Geometry: final body of the model. Coordinates: model frame, mm. A direction names the side the tool comes from. Give positions to 0.01 mm unless a question says otherwise; leave off trailing zeros. Write each loop counter-clockwise with the first axis right and the second up, starting at its lowest first coordinate (ties: lowest second). Pieces come first, ordered by that corner, then holes. Notation, with made-up numbers: (19, 4) -> (70, 4) arc R27 cw to (70, 38) -> close; hole circle Ø3 at (33.25, 59). An arc over 180 degrees is marked (long way). Answer in a Markdown table with one row per item. Add a question column.
from build123d import *

# Parameters (mm, degrees)
F0_R     = 1.5
F1_DEPTH = 5
F2_R     = 5


# Not quite as in the source:
# - a feature names something its author has since deleted; it is built from what else it names


with BuildPart() as f1:
    # F0 (on Top) → F1 (new body)
    with BuildSketch(Plane.XY):
        with BuildLine():
            Line((32, -25.9806431703), (45.0002060157, -25.9806431703))
            Line((45.0002060157, -25.9806431703), (34.8648160141, -8.425632733))
            ThreePointArc((34.8648160141, -8.425632733), (33.2306953855, -12.3086021935), (31.1657699329, -15.9806431703))
            Line((31.1657699329, -15.9806431703), (32, -15.9806431703))
            Line((32, -15.9806431703), (32, -25.9806431703))
        make_face()
        with BuildLine():
            Line((34.8648160141, -8.425632733), (45.0002060157, -25.9806431703))
            ThreePointArc((45.0002060157, -25.9806431703), (42.4187903028, 24.4905), (0.0002060157, 51.9616431703))
            Line((0.0002060157, 51.9616431703), (6.7047123911, 40.3490974884))
            ThreePointArc((6.7047123911, 40.3490974884), (28.4347881869, 27.6357391565), (37, 3.9616431703))
            ThreePointArc((37, 3.9616431703), (36.4622969142, -2.3233312719), (34.8648160141, -8.425632733))
        make_face()
        with Locations((41.2026322213, 9.0961922878)):
            Circle(F0_R, mode=Mode.SUBTRACT)
        with Locations((25.2027902051, 36.8090964203)):
            Circle(F0_R, mode=Mode.SUBTRACT)
        with BuildLine():
            Line((32, -55.9806431703), (32, -25.9806431703))
            Line((32, -25.9806431703), (21.7361332508, -25.9806431703))
            ThreePointArc((21.7361332508, -25.9806431703), (0, -33.0383568297), (-21.7361332508, -25.9806431703))
            Line((-21.7361332508, -25.9806431703), (-32, -25.9806431703))
            Line((-32, -25.9806431703), (-32, -55.9806431703))
            Line((-32, -55.9806431703), (32, -55.9806431703))
        make_face()
        with Locations((-16, -50.8592247836)):
            Circle(F0_R, mode=Mode.SUBTRACT)
        with Locations((-24.9, -29.9806431703)):
            Circle(F0_R, mode=Mode.SUBTRACT)
        with Locations((16, -50.9806431703)):
            Circle(F0_R, mode=Mode.SUBTRACT)
        with Locations((24.9, -29.9806431703)):
            Circle(F0_R, mode=Mode.SUBTRACT)
        with BuildLine():
            Line((21.7361332508, -25.9806431703), (32, -25.9806431703))
            Line((32, -25.9806431703), (32, -15.9806431703))
            Line((32, -15.9806431703), (31.1657699329, -15.9806431703))
            ThreePointArc((31.1657699329, -15.9806431703), (26.9193766665, -21.422350997), (21.7361332508, -25.9806431703))
        make_face()
        with BuildLine():
            Line((6.7047123911, 40.3490974884), (0.0002060157, 51.9616431703))
            Line((0.0002060157, 51.9616431703), (-6.7042513108, 40.3491824435))
            ThreePointArc((-6.7042513108, 40.3491824435), (0.0002344208, 40.9616431696), (6.7047123911, 40.3490974884))
        make_face()
        with BuildLine():
            Line((-6.7042513108, 40.3491824435), (0.0002060157, 51.9616431703))
            ThreePointArc((0.0002060157, 51.9616431703), (-42.4183782713, 24.4905), (-44.9997939843, -25.9806431703))
            Line((-44.9997939843, -25.9806431703), (-34.8646590472, -8.4260745178))
            ThreePointArc((-34.8646590472, -8.4260745178), (-32.04293994, 22.4616431703), (-6.7042513108, 40.3491824435))
        make_face()
        with Locations((-41.202520651, 9.0964271731)):
            Circle(F0_R, mode=Mode.SUBTRACT)
        with Locations((-25.202520651, 36.8092400942)):
            Circle(F0_R, mode=Mode.SUBTRACT)
        with BuildLine():
            ThreePointArc((-21.7361332508, -25.9806431703), (0, -33.0383568297), (21.7361332508, -25.9806431703))
            Line((21.7361332508, -25.9806431703), (-21.7361332508, -25.9806431703))
        make_face()
        with BuildLine():
            Line((-21.7361332508, -25.9806431703), (21.7361332508, -25.9806431703))
            ThreePointArc((21.7361332508, -25.9806431703), (26.9193766665, -21.422350997), (31.1657699329, -15.9806431703))
            Line((31.1657699329, -15.9806431703), (-31.1657699329, -15.9806431703))
            ThreePointArc((-31.1657699329, -15.9806431703), (-26.9193766665, -21.422350997), (-21.7361332508, -25.9806431703))
        make_face()
        with BuildLine():
            Line((-34.8646590472, -8.4260745178), (-44.9997939843, -25.9806431703))
            Line((-44.9997939843, -25.9806431703), (-32, -25.9806431703))
            Line((-32, -25.9806431703), (-32, -15.9806431703))
            Line((-32, -15.9806431703), (-31.1657699329, -15.9806431703))
            ThreePointArc((-31.1657699329, -15.9806431703), (-33.2305923015, -12.3088127328), (-34.8646590472, -8.4260745178))
        make_face()
        with BuildLine():
            Line((-32, -25.9806431703), (-21.7361332508, -25.9806431703))
            ThreePointArc((-21.7361332508, -25.9806431703), (-26.9193766665, -21.422350997), (-31.1657699329, -15.9806431703))
            Line((-31.1657699329, -15.9806431703), (-32, -15.9806431703))
            Line((-32, -15.9806431703), (-32, -25.9806431703))
        make_face()
    extrude(amount=F1_DEPTH)

    # F2
    f2_edges = [f1.edges().sort_by_distance(p)[0] for p in [
        (-32, -25.980643, 2.5),
        (-44.999794, -25.980643, 2.5),
        (32, -25.980643, 2.5),
        (45.000206, -25.980643, 2.5),
        (-32, -55.980643, 2.5),
        (32, -55.980643, 2.5),
        (-31.16577, -15.980643, 2.5),
        (31.16577, -15.980643, 2.5),
    ]]
    fillet(f2_edges, radius=F2_R)


solid = f1.part
Q1. Section D-D on x = -5. Return loops of the section in (y, z), and give its area (3 significant figures).
Q2. Section C-C on z = 0.9. Count the separate pieces of the cut face and the enclosed holes in it, and give its area (3 significant figures).
Q3. Contact query for flat-ended pins moving along their axis: pin 1 Ø3 at (y, z) = (10, 1) entering from +X; pin 2 Ø2 at (x, z) = (12, 3) entering from +Y; pin 3 Ø2 at (x, z) = (26.5, 1) entering from +Y. Output: stop coordinate, or through.
Q4. Section B-B on x = -16. Return loops of the section in (y, z).
Q5. Access query for faces 1 (the flat face through (-39, -25.981, 2)), 2 (the flat face through (-1, -25, 0)), 3 (the cylindrical face through (30.85, -15.28, 2.54)), 4 (the flat face through (32, -41, 2)), 5 (the cylindrical face through (-41.139, 26.598, 2.465)). Directions: +Z, -Z, +X, -X, +Y, -Y. A direction counts if a zero-diameter tool reaches every point of the face in a straight line with its end or side. Return the directions, or none.
Q6. Section A-A on y = 19.5. Return loops of the section in (x, z), and give its area (3 significant figures).
Q7. Pull-direction query (X, two-part tool) for faces 6 (the flat face through (39, -25.981, 2)), 7 (the cylindrical face through (33.43, -27.48, 2.54)), 8 (the cylindrical face through (25.008, 38.296, 2.465)); classes: +X half, -X half, draft (parallel to the pull), parting line (faces both ways), or undercut.
Q8. Line query: probe 1 along Y at (x, z) = (-24.9, 3.25); probe 2 along X at (y, z) = (-13, 0.9); probe 3 along Y at (x, z) = (-16, 2.6). Output: solid intervals per line, ascending. Write a range as from..to.
Checks:
| question | item | result |
|---|---|---|
| 1 | outline | (-55.98, 0) -> (-15.98, 0) -> (-15.98, 5) -> (-55.98, 5) -> close; (40.62, 0) -> (51.22, 0) -> (51.22, 5) -> (40.62, 5) -> close |
| 1 | area | 253 mm^2 |
| 2 | separate pieces | 1 |
| 2 | enclosed holes | 9 |
| 2 | area | 4,720 mm^2 |
| 3 | pin 1 | x = 48.6 |
| 3 | pin 2 | y = 49.69 |
| 3 | pin 3 | y = 42.68 |
| 4 | outline | (-55.98, 0) -> (-52.36, 0) -> (-52.36, 5) -> (-55.98, 5) -> close; (-49.36, 0) -> (-15.98, 0) -> (-15.98, 5) -> (-49.36, 5) -> close; (37.32, 0) -> (47.85, 0) -> (47.85, 5) -> (37.32, 5) -> close |
| 5 | face 1 | +Z, -Z, -X, -Y |
| 5 | face 2 | -Z, +X, -X, +Y, -Y |
| 5 | face 3 | +Z, -Z |
| 5 | face 4 | +Z, -Z, +X, -Y |
| 5 | face 5 | +Z, -Z, -X |
| 6 | outline | (-44.97, 0) -> (-33.58, 0) -> (-33.58, 5) -> (-44.97, 5) -> close; (33.58, 0) -> (44.97, 0) -> (44.97, 5) -> (33.58, 5) -> close |
| 6 | area | 114 mm^2 |
| 7 | face 6 | draft |
| 7 | face 7 | +X half |
| 7 | face 8 | undercut |
| 8 | probe 1 | -55.98..-31.48, -28.48..-15.98, 31.33..35.34, 38.28..43.08 |
| 8 | probe 2 | -49..-32.88, 32.88..49 |
| 8 | probe 3 | -55.98..-52.36, -49.36..-15.98, 37.32..47.85 |
